Answer from the drawing. Dimensions are ordinates in mm from the lowest x, y and z of the part. A direction names the side the tool comes from. Give positions to 0.01 mm unless a question says otherwise; leave off trailing zeros. Order: outer loops, then holes, each group sorted by start corner. A loop starts at its lowest first (then second) coordinate and runs counter-clockwise, first axis right, second up. Notation, with made-up numbers: (87, 9) - (142, 9) arc R15 ccw to (142, 19) - close; hole circle Ø9 at (81, -15). An arc over 180 degrees is marked (long way). Answer in a Markdown table with one row per item.
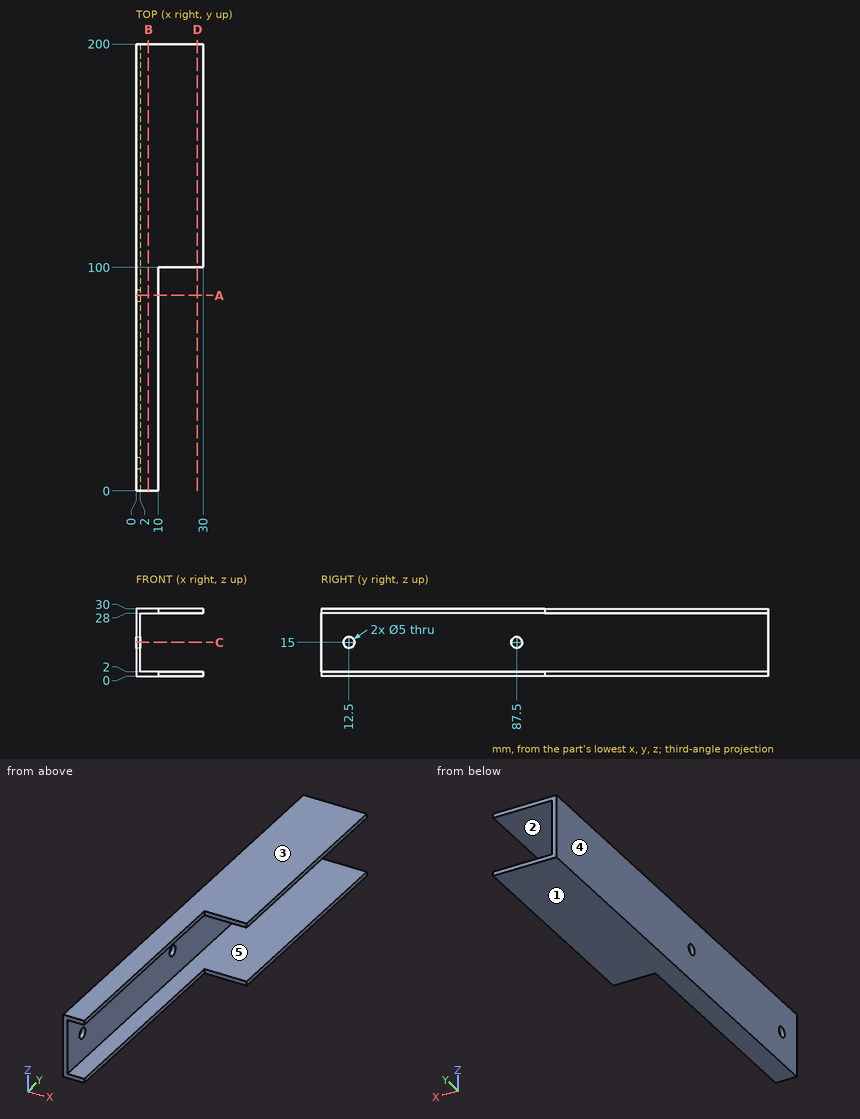
Item 1: Find section C-C on z = 15. Write down the section's boundary in (x, y).
Answer block:
| item | result |
|---|---|
| outline | (0, 0) - (2, 0) - (2, 10) - (0, 10) - close; (0, 15) - (2, 15) - (2, 85) - (0, 85) - close; (0, 90) - (2, 90) - (2, 200) - (0, 200) - close |
Item 2: Find section A-A on y = 87.5. Write down the section's boundary in (x, z).
Answer block:
| item | result |
|---|---|
| outline | (0, 0) - (10, 0) - (10, 2) - (2, 2) - (2, 12.5) - (0, 12.5) - close; (0, 17.5) - (2, 17.5) - (2, 28) - (10, 28) - (10, 30) - (0, 30) - close |
Item 3: Find section B-B on x = 5.5. Write down the section's boundary in (y, z).
Answer block:
| item | result |
|---|---|
| outline | (0, 0) - (200, 0) - (200, 2) - (0, 2) - close; (0, 28) - (200, 28) - (200, 30) - (0, 30) - close |
Item 4: Determine the mould class of the marked faces 3, 4 and 5 for opening direction Z: pulls with the +Z half, pulls with the -Z half, needs draft (parallel to the pull), parting line crosses it, or undercut.
Answer block:
| item | result |
|---|---|
| face 3 | pulls with the +Z half |
| face 4 | needs draft |
| face 5 | undercut |
Item 5: Which of the six approach directions +Z, -Z, +X, -X, +Y, -Y give full straight-line access (tool end or side, diameter ignored) to the marked faces 1 and 2?
Answer block:
| item | result |
|---|---|
| face 1 | -Z, +X, -X, +Y, -Y |
| face 2 | +X, +Y, -Y |
Item 6: Consider line 1 (Y direction, x = 0.4, z = 15); line 2 (Z direction, x = 22, y = 176.5); line 3 (Z direction, x = 0.6, y = 12.5). Determine where each line is inside the solid, lowest interval first.
Answer block:
| item | result |
|---|---|
| line 1 | 0 to 10, 15 to 85, 90 to 200 |
| line 2 | 0 to 2, 28 to 30 |
| line 3 | 0 to 12.5, 17.5 to 30 |
Item 7: Find section D-D on x = 27.5. Write down the section's boundary in (y, z).
Answer block:
| item | result |
|---|---|
| outline | (100, 0) - (200, 0) - (200, 2) - (100, 2) - close; (100, 28) - (200, 28) - (200, 30) - (100, 30) - close |
Item 8: Each of these flat-tipped pins is pushed along its axis until it touches: P1, Ø4, axis at y = 113, z = 11, coming from the +X side; P2, Ø1, axis at y = 40.5, z = 0.5, coming from the +X side; P3, Ø4.5, axis at y = 87.5, z = 15, coming from the -X side; P4, Ø2, axis at x = 19, z = 29.5, coming from the -Y side. Where does it stop, or does it pass through?
Answer block:
| item | result |
|---|---|
| P1 | x = 2 |
| P2 | x = 10 |
| P3 | through |
| P4 | y = 100 |
